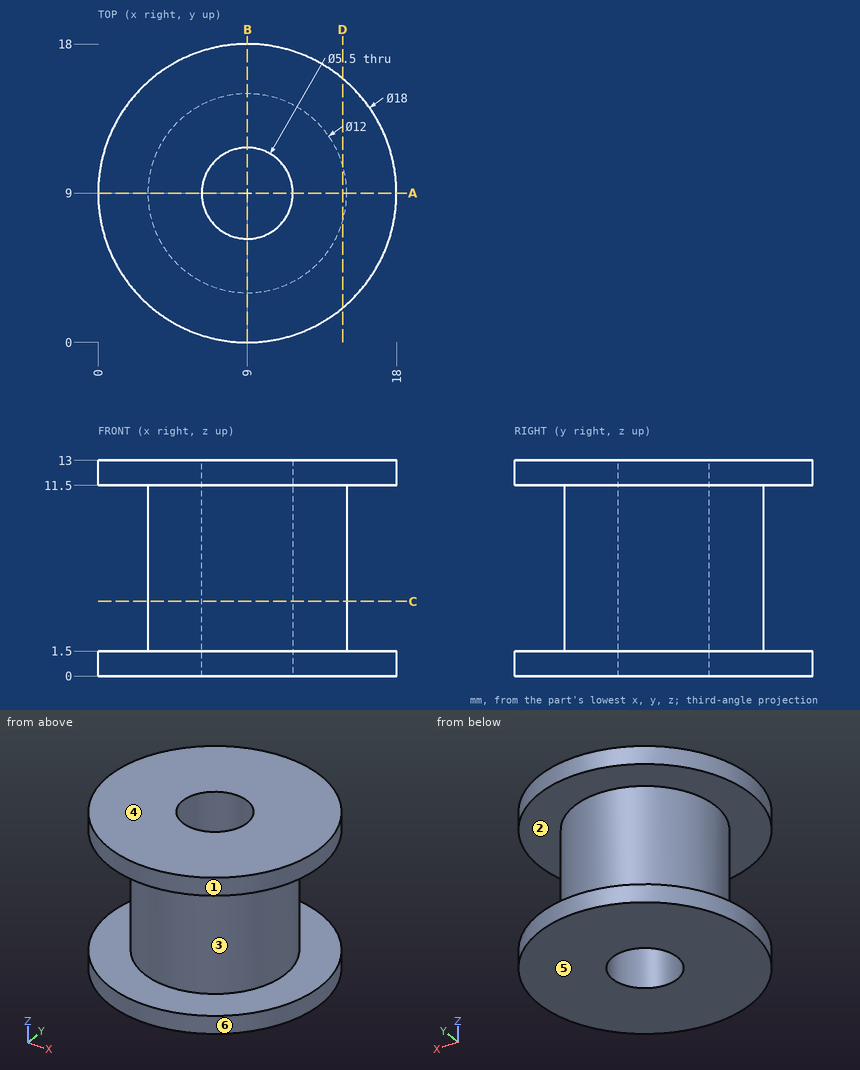
Geometry check sheet. Reference: drawing and pictorial views, mm from the part's lowest x, y, z. A direction names the side the tool comes from. Round coordinates to 2 decimals unless told otherwise and drop trailing zeros. Loops run counter-clockwise (first coordinate to the right, second up) from the corner with the lowest first, then second, coordinate; pieces in that order, holes last. Notation, with made-up numbers: M 5,47 L 64,47 A17 cw 64,55 Z; hole C 77.5,58.25 d2. An arc over 180 degrees is marked long. Return JSON: item names as keys, results as strings. Group by question number.
(1) Section check C-C, the plane z = 4.5. Enter the section's corners in (x, y), and give its area (3 significant figures).
(2) Go/stop test with flat-tipped pins: pin 1 (1 mm diameter, centred on y = 12.5, z = 7, fed in from -X); pin 2 (5 mm diameter, centred on x = 9, y = 9, fed in from +Z). Record where each tip stops, or that it passes through.
(3) Mould release check, pull along Z, two halves, no side actions. Record for the marked faces 3, 4, 5 and 6: pulls with the +Z half, pulls with the -Z half, needs draft (parallel to the pull), parting line crosses it, or undercut.
(4) Section check A-A, the plane y = 9. Enter the section's corners in (x, z).
(5) Scan lines: line 1 along Y through (x, z) = (9, 9.5); line 2 along Z through (x, y) = (15, 6.75); line 3 along Y through (x, z) = (7.25, 5). Record each from-to range of solid material in increasing order. Write a range as [from, to].
(6) Set-up check for the marked faces 1 and 2: record each of +Z, -Z, +X, -X, +Y, -Y from which the full face is reachable in a straight line by a thin tool's end or side.
(7) Section check D-D, the plane x = 14.75. Enter the section's corners in (y, z), and give its area (3 significant figures).
Data:
{
 "1": {"outline": "C 9,9 d12; hole C 9,9 d5.5", "area": "89.3 mm²"},
 "2": {"pin 1": "x = 3.8", "pin 2": "through"},
 "3": {"face 3": "undercut", "face 4": "pulls with the +Z half", "face 5": "pulls with the -Z half", "face 6": "needs draft"},
 "4": {"outline": "M 0,0 L 6.25,0 L 6.25,13 L 0,13 L 0,11.5 L 3,11.5 L 3,1.5 L 0,1.5 Z; M 11.75,0 L 18,0 L 18,1.5 L 15,1.5 L 15,11.5 L 18,11.5 L 18,13 L 11.75,13 Z"},
 "5": {"line 1": "[3, 6.25], [11.75, 15]", "line 2": "[0, 1.5], [11.5, 13]", "line 3": "[3.26, 6.88], [11.12, 14.74]"},
 "6": {"face 1": "+Z, -Z", "face 2": "none"},
 "7": {"outline": "M 2.08,0 L 15.92,0 L 15.92,1.5 L 10.71,1.5 L 10.71,11.5 L 15.92,11.5 L 15.92,13 L 2.08,13 L 2.08,11.5 L 7.29,11.5 L 7.29,1.5 L 2.08,1.5 Z", "area": "75.8 mm²"}
}
